from build123d import *

# Parameters (mm, degrees)
EXTRUDE_1_DEPTH          = 40
CUT_EXTRUDE_1_DEPTH      = 42.569219382
CUT_EXTRUDE_1_DEPTH_BACK = 42.569219382
CUT_EXTRUDE_START        = -4
SKETCH_5_R               = 8
CUT_EXTRUDE_2_DEPTH      = 4
SKETCH_6_R               = 8
CUT_EXTRUDE_3_DEPTH      = 4
CUT_EXTRUDE_4_DEPTH      = 100
CUT_EXTRUDE_5_DEPTH      = 100


with BuildPart() as part:
    # 草图2 → 凸台-拉伸1 (new body)
    with BuildSketch(Plane(origin=(0, 0, 0), x_dir=(1, 0, 0), z_dir=(0, 1, 0))):
        Polygon((8, 3.313708499), (3.313708499, 8), (-3.313708499, 8), (-8, 3.313708499), (-8, -3.313708499), (-3.313708499, -8), (3.313708499, -8), (8, -3.313708499), align=None)
    extrude(amount=EXTRUDE_1_DEPTH)

    # 草图4 → 切除-拉伸1 (cut, two sides: drawn at the far end of the back side and taken through both)
    with BuildSketch(Plane.XY.offset(-CUT_EXTRUDE_1_DEPTH_BACK)):
        with BuildLine():
            Line((-8, 8), (-8, -3.683086278))
            Line((-8, -3.683086278), (8, -3.683086278))
            Line((8, -3.683086278), (8, 8))
            ThreePointArc((8, 8), (0, 0), (-8, 8))
        make_face()
    extrude(amount=CUT_EXTRUDE_1_DEPTH + CUT_EXTRUDE_1_DEPTH_BACK, mode=Mode.SUBTRACT)

    # 草图5 → 切除-拉伸2 (cut)
    with BuildSketch(Plane.XY.offset(8).offset(CUT_EXTRUDE_START)):
        with Locations((0, 8)):
            Circle(SKETCH_5_R)
    extrude(amount=CUT_EXTRUDE_2_DEPTH, mode=Mode.SUBTRACT)

    # 草图6 → 切除-拉伸3 (cut)
    with BuildSketch(Plane(origin=(0, 0, -8), x_dir=(-1, 0, 0), z_dir=(0, 0, -1))):
        with Locations((0, 8)):
            Circle(SKETCH_6_R)
    extrude(amount=-CUT_EXTRUDE_3_DEPTH, mode=Mode.SUBTRACT)

    # 草图7 → 切除-拉伸4 (cut)
    with BuildSketch(Plane(origin=(0, 0, -8), x_dir=(-1, 0, 0), z_dir=(0, 0, -1))):
        with BuildLine():
            Line((-8, 32), (-8, 48.980650176))
            Line((-8, 48.980650176), (8, 48.980650176))
            Line((8, 48.980650176), (8, 32))
            ThreePointArc((8, 32), (0, 40), (-8, 32))
        make_face()
    extrude(amount=-CUT_EXTRUDE_4_DEPTH, mode=Mode.SUBTRACT)

    # 草图8 → 切除-拉伸5 (cut)
    with BuildSketch(Plane.ZY.offset(8)):
        with BuildLine():
            Line((-8, 32), (-8, 42.16921849))
            Line((-8, 42.16921849), (8, 42.16921849))
            Line((8, 42.16921849), (8, 32))
            ThreePointArc((8, 32), (0, 40), (-8, 32))
        make_face()
    extrude(amount=-CUT_EXTRUDE_5_DEPTH, mode=Mode.SUBTRACT)


solid = part.part
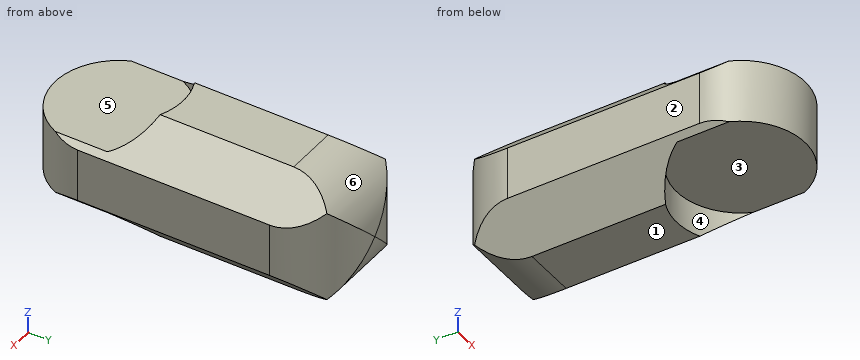
Geometry: final body of the model. Coordinates: model frame, mm. Face numbers are marked on the shaded views. A direction names the side the tool comes from. Round coordinates to 2 decimals unless told otherwise and drop trailing zeros. Loops run counter-clockwise (first coordinate to the right, second up) from the corner with the lowest first, then second, coordinate; pieces in that order, holes last.
Q1. Material intervals for L1, parallel to X at y = 17.5, z = 4; L2, parallel to X at y = 33.5, z = -2; L3, parallel to Y at x = 2.75, z = 3.5, sorted ascending.
Q2. Pull-direction query (X, two-part tool) for the marked faces 1, 2 and 3; classes: released by +X, released by -X, zero draft, split by the parting line, or undercut.
Q3. Pin query (flat end, axial travel): P1, Ø1, axis at y = 25.5, z = 5, coming from the +X side; P2, Ø1, axis at y = 25.5, z = -6, coming from the +X side; P3, Ø4.5, axis at x = 2.5, y = 11, coming from the +Z side. Return the tip coordinate at first contact, or that it passes through.
Q4. Section B-B on x = -0.5. Return loops of the section in (y, z), plus the area to 3 significant figures.
Q5. Access query for the marked faces 4, 5 and 6. Directions: +Z, -Z, +X, -X, +Y, -Y. A direction counts if a zero-diameter tool reaches every point of the face in a straight line with its end or side. Return the directions, or none.
Q6. Section C-C on x = 4.5. Return loops of the section in (y, z), plus the area to 3 significant figures.
Q7. Section A-A on y = 27. Return loops of the section in (x, z), plus the area to 3 significant figures.
Q8. Section D-D on z = 6.5. Return loops of the section in (x, y), plus the area to 3 significant figures.
Evaluation:
1. L1: x = -7.31 to 7.31
1. L2: x = -7.86 to 7.86
1. L3: y = 0.49 to 39.19
2. face 1: zero draft
2. face 2: released by -X
2. face 3: undercut
3. P1: stops at x = 6.81
3. P2: stops at x = 5.81
3. P3: stops at z = 4
4. outline: (0.02, -4) - (15.98, -4) - (15.98, -8) - (32, -8) arc R8 ccw to (39.98, -0.5) - (39.98, 0.5) arc R8 ccw to (32, 8) - (15.98, 8) - (15.98, 4) - (0.02, 4) - close
4. area: 485 mm2
5. face 4: -Z, -Y
5. face 5: +Z, -Y
5. face 6: +Z, +X, -X, +Y
6. outline: (1.39, -4) - (14.61, -4) - (14.61, -6.81) - (36.19, -6.81) arc R8 ccw to (38.61, -4.5) - (38.61, 4.5) arc R8 ccw to (36.19, 6.81) - (14.61, 6.81) - (14.61, 4) - (1.39, 4) - close
6. area: 428 mm2
7. outline: (-8, -3.31) - (-3.31, -8) - (3.31, -8) - (8, -3.31) - (8, 3.31) - (3.31, 8) - (-3.31, 8) - (-8, 3.31) - close
7. area: 212 mm2
8. outline: (-4.81, 14.39) arc R8 cw to (4.81, 14.39) - (4.81, 36.66) - (-4.81, 36.66) - close
8. area: 204 mm2
